Input: part model. Units: mm. Frame: model coordinates. Face numbers are marked on the shaded views. A direction names the side the tool comes from. Give positions to 0.01 mm unless a question says otherwise; leave off trailing zeros. Loops run counter-clockwise (first coordinate to the right, second up) from the corner with the lowest first, then second, coordinate; pieces in that order, holes last. Notation, with made-up numbers: (9, 31.5) -> (54, 31.5) arc R31 ccw to (54, 61.5) -> close; hole circle Ø10 at (29.5, -24.75). An arc over 180 degrees is marked (long way). Answer as a JSON object with one key per item and string values.
```python
from build123d import *

# Parameters (mm, degrees)
CUT_EXTRUDE1_DEPTH      = 15
CUT_EXTRUDE1_DEPTH_BACK = 15
SKETCH2_R               = 2.25
SKETCH3_W               = 20
SKETCH3_H               = 10
CUT_EXTRUDE2_DEPTH      = 40


with BuildPart() as part:
    # Sketch1 → Revolve1 (revolve)
    with BuildSketch(Plane.XY):
        with BuildLine():
            Line((0, 0), (0, 40))
            Line((0, 40), (15, 40))
            Line((15, 40), (15, -47.696960071))
            Line((15, -47.696960071), (15, -97.696960071))
            ThreePointArc((15, -97.696960071), (-34.420886291, -55.284845035), (0, 0))
        make_face()
    revolve(axis=Axis((15, 40, 0), (0, -1, 0)))

    # Sketch2 → Cut-Extrude1 (cut, two sides: drawn at the far end of the back side and taken through both)
    with BuildSketch(Plane.XY.offset(-CUT_EXTRUDE1_DEPTH_BACK)):
        with Locations(Location((15, 30, 0), (0, 0, 180))):
            Circle(SKETCH2_R)
        with Locations(Location((15, 20, 0), (0, 0, 180))):
            Circle(SKETCH2_R)
        with Locations(Location((15, 10, 0), (0, 0, 180))):
            Circle(SKETCH2_R)
    extrude(amount=CUT_EXTRUDE1_DEPTH + CUT_EXTRUDE1_DEPTH_BACK, mode=Mode.SUBTRACT)

    # Sketch3 → Cut-Extrude2 (cut)
    with BuildSketch(Plane(origin=(0, 40, 0), x_dir=(1, 0, 0), z_dir=(0, 1, 0))):
        with Locations((15, 0)):
            Rectangle(SKETCH3_W, SKETCH3_H)
    extrude(amount=-CUT_EXTRUDE2_DEPTH, mode=Mode.SUBTRACT)


solid = part.part
```
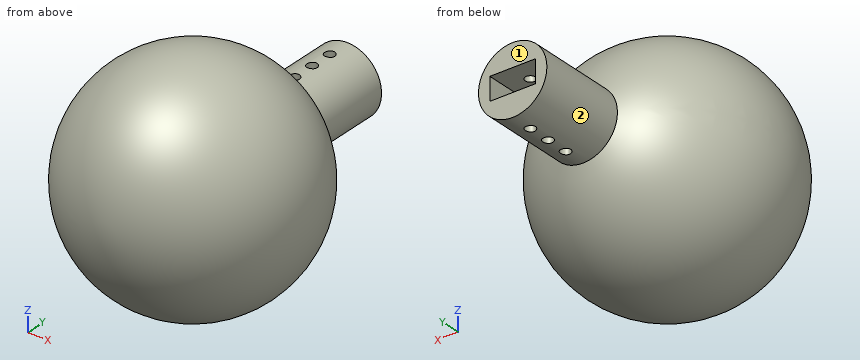
Q1. Ray query, line 1 along Y through (x, z) = (15, -12.5); line 2 along Y through (x, z) = (15, -11); line 3 along X through (y, z) = (30, 12). Return the intervals inside material, ascending.
Evaluation:
{"line 1": "y = -96.11 to 7.75, 12.25 to 17.75, 22.25 to 27.75, 32.25 to 40", "line 2": "y = -96.47 to 7.75, 12.25 to 17.75, 22.25 to 27.75, 32.25 to 40", "line 3": "x = 6 to 12.75, 17.25 to 24"}
Q2. Section B-B, the plane y = 16. Return the cut outline in (x, z), then the cut area to 3 significant figures.
Evaluation:
{"outline": "circle Ø30 at (15, 0); hole (5, -5) -> (25, -5) -> (25, 5) -> (5, 5) -> close", "area": "507 mm2"}
Q3. Access query for the marked faces 1 and 2. Directions: +Z, -Z, +X, -X, +Y, -Y. A direction counts if a zero-diameter tool reaches every point of the face in a straight line with its end or side. Return the directions, or none.
Evaluation:
{"face 1": "+Z, -Z, +X, -X, +Y", "face 2": "+Y"}
Q4. Section A-A, the plane x = 15. Give the number of separate pieces and of enclosed holes in the cut face, then the cut area to 3 significant figures.
Evaluation:
{"separate pieces": "7", "enclosed holes": "0", "area": "8,340 mm2"}
Q5. Section C-C, the plane z = 0. Return the cut outline in (x, y).
Evaluation:
{"outline": "(0, 0) arc R50 ccw (long way) to (30, 0) -> (30, 40) -> (25, 40) -> (25, 0) -> (5, 0) -> (5, 40) -> (0, 40) -> close"}
Q6. Pin query (flat end, axial travel): pin 1 (11 mm diameter, centred on y = 19.5, z = 1.5, fed in from -X); pin 2 (2 mm diameter, centred on y = -64, z = -2, fed in from +X); pin 3 (1 mm diameter, centred on x = 1, z = -2, fed in from -Y); pin 4 (3.5 mm diameter, centred on x = 15, y = 30, fed in from +Z). Return the tip coordinate at first contact, or that it passes through.
Evaluation:
{"pin 1": "stops at x = 0", "pin 2": "stops at x = 62.56", "pin 3": "stops at y = -95.8", "pin 4": "passes through"}
Q7. Section D-D, the plane y = 30. Return the cut outline in (x, z), then the cut area to 3 significant figures.
Evaluation:
{"outline": "(5, -5) -> (5, 5) -> (12.75, 5) -> (12.75, 14.83) arc R15 ccw to (12.75, -14.83) -> (12.75, -5) -> close; (17.25, -14.83) arc R15 ccw to (17.25, 14.83) -> (17.25, 5) -> (25, 5) -> (25, -5) -> (17.25, -5) -> close", "area": "417 mm2"}
